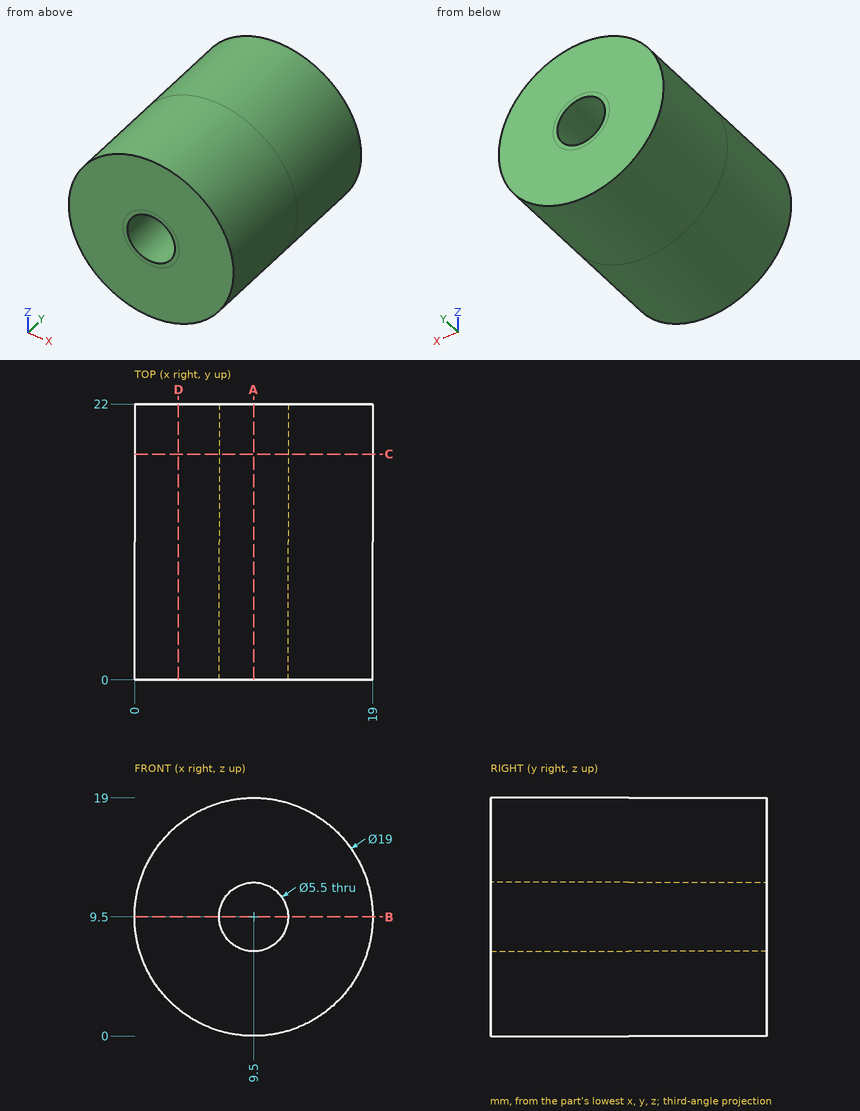
Drawing for the job (mm, zero at the part's lowest x, y, z). Coordinates: 2 decimals unless noted, no trailing zeros. Order: outer loops, then holes, each group sorted by start corner. A loop starts at its lowest first (then second) coordinate and runs counter-clockwise, first axis right, second up. Notation, with made-up numbers: (-32.5, 72.5) - (10.5, 72.5) arc R32 cw to (10.5, 98.5) - close; hole circle Ø1 at (74.25, 86). An arc over 180 degrees is marked (long way). Use a Markdown table: item, result. Add a question column.
(1) Saw through at C-C (y = 18). Give the cut face in (x, z), then the cut area to 3 significant figures.
(2) Saw through at B-B (z = 9.5). Give the cut face in (x, y), then the cut area to 3 significant figures.
(3) Saw through at D-D (x = 3.5). Give the cut face in (y, z).
(4) Saw through at A-A (x = 9.5). Give the cut face in (y, z), then the cut area to 3 significant figures.
(5) Flat gauge pins, fed straight in: pin 1 (5 mm diameter, centred on x = 12.5, y = 17, fed in from -Z); pin 2 (5 mm diameter, centred on y = 11, z = 14.5, fed in from +X); pin 3 (1.5 mm diameter, centred on y = 3.5, z = 12.5, fed in from -X). Where does each tip first touch, or does it go through?
(6) Drill centre lines: line 1 along X through (y, z) = (6.25, 9.5); line 2 along Z through (x, y) = (11.25, 9.75); line 3 along X through (y, z) = (5.25, 7.5). Where is each one in solid material? Low to high. Write a range as [from, to].
Solved:
| question | item | result |
|---|---|---|
| 1 | outline | circle Ø19 at (9.5, 9.5); hole circle Ø5.5 at (9.5, 9.5) |
| 1 | area | 260 mm² |
| 2 | outline | (0, 0) - (6.75, 0) - (6.75, 22) - (0, 22) - close; (12.25, 0) - (19, 0) - (19, 22) - (12.25, 22) - close |
| 2 | area | 297 mm² |
| 3 | outline | (0, 2.13) - (22, 2.13) - (22, 16.87) - (0, 16.87) - close |
| 4 | outline | (0, 0) - (22, 0) - (22, 6.75) - (0, 6.75) - close; (0, 12.25) - (22, 12.25) - (22, 19) - (0, 19) - close |
| 4 | area | 297 mm² |
| 5 | pin 1 | stops at z = 0.01 |
| 5 | pin 2 | stops at x = 18.67 |
| 5 | pin 3 | stops at x = 0.27 |
| 6 | line 1 | x = [0, 6.75], [12.25, 19] |
| 6 | line 2 | z = [0.16, 7.38], [11.62, 18.84] |
| 6 | line 3 | x = [0.21, 7.61], [11.39, 18.79] |
